Work out the finished part from the listing and answer in its coordinate system (mm). Round coordinates to 2 decimals unless told otherwise and drop trailing zeros. Write each loop counter-clockwise with the first axis right and the second up, starting at its lowest first coordinate (ties: lowest second). Pieces come first, ordered by that corner, then holes.
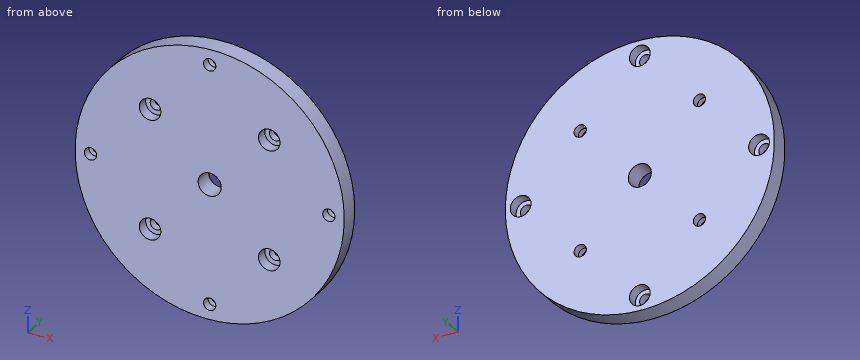
from build123d import *

# Parameters (mm, degrees)
SKETCH1_R           = 35
SKETCH1_R_2         = 3
BOSS_EXTRUDE1_DEPTH = 5
SKETCH2_R           = 1.6
CUT_EXTRUDE1_DEPTH  = 5
SKETCH4_R           = 2.8
SKETCH4_R_2         = 1.6
CUT_EXTRUDE2_DEPTH  = 3
SKETCH5_R           = 1.6
CUT_EXTRUDE3_DEPTH  = 10
SKETCH6_R           = 2.7
CUT_EXTRUDE4_DEPTH  = 2.8


with BuildPart() as part:
    # Sketch1 → Boss-Extrude1 (new body)
    with BuildSketch(Plane(origin=(0, 0, 0), x_dir=(1, 0, 0), z_dir=(0, 1, 0))):
        Circle(SKETCH1_R)
        Circle(SKETCH1_R_2, mode=Mode.SUBTRACT)
    extrude(amount=BOSS_EXTRUDE1_DEPTH)

    # Sketch2 → Cut-Extrude1 (cut)
    with BuildSketch(Plane.XZ):
        with Locations((15.5, 15.5)):
            Circle(SKETCH2_R)
        with Locations((15.5, -15.5)):
            Circle(SKETCH2_R)
        with Locations((-15.5, -15.5)):
            Circle(SKETCH2_R)
        with Locations((-15.5, 15.5)):
            Circle(SKETCH2_R)
    extrude(amount=-CUT_EXTRUDE1_DEPTH, mode=Mode.SUBTRACT)

    # Sketch4 → Cut-Extrude2 (cut)
    with BuildSketch(Plane.XZ):
        with Locations((-15.5, 15.5)):
            Circle(SKETCH4_R)
        with Locations((-15.5, 15.5)):
            Circle(SKETCH4_R_2, mode=Mode.SUBTRACT)
        with Locations((15.5, 15.5)):
            Circle(SKETCH4_R)
        with Locations((15.5, 15.5)):
            Circle(SKETCH4_R_2, mode=Mode.SUBTRACT)
        with Locations((15.5, -15.5)):
            Circle(SKETCH4_R)
        with Locations((15.5, -15.5)):
            Circle(SKETCH4_R_2, mode=Mode.SUBTRACT)
        with Locations((-15.5, -15.5)):
            Circle(SKETCH4_R)
        with Locations((-15.5, -15.5)):
            Circle(SKETCH4_R_2, mode=Mode.SUBTRACT)
    extrude(amount=-CUT_EXTRUDE2_DEPTH, mode=Mode.SUBTRACT)

    # Sketch5 → Cut-Extrude3 (cut)
    with BuildSketch(Plane(origin=(0, 5, 0), x_dir=(1, 0, 0), z_dir=(0, 1, 0))):
        with Locations((0, 31)):
            Circle(SKETCH5_R)
        with Locations((31, 0)):
            Circle(SKETCH5_R)
        with Locations((0, -31)):
            Circle(SKETCH5_R)
        with Locations((-31, 0)):
            Circle(SKETCH5_R)
    extrude(amount=-CUT_EXTRUDE3_DEPTH, mode=Mode.SUBTRACT)

    # Sketch6 → Cut-Extrude4 (cut)
    with BuildSketch(Plane(origin=(0, 5, 0), x_dir=(1, 0, 0), z_dir=(0, 1, 0))):
        with Locations((0, 31)):
            Circle(SKETCH6_R)
        with Locations((31, 0)):
            Circle(SKETCH6_R)
        with Locations((0, -31)):
            Circle(SKETCH6_R)
        with Locations((-31, 0)):
            Circle(SKETCH6_R)
    extrude(amount=-CUT_EXTRUDE4_DEPTH, mode=Mode.SUBTRACT)


solid = part.part
Q1. Find the intervals of material crossed by L1, parallel to Z at x = 0, y = 0.7; L2, parallel to Z at x = 0, y = 3.3; L3, parallel to Z at x = 16, y = 4.1, in increasing order.
Q2. Find section B-B (y = 3.8). Count the separate pieces of the cut face and the enclosed holes in it, plus the area to 3 significant figures.
Q3. Given pin 1 (1.5 mm diameter, centred on x = 8, y = 4, fed in from -Z); pin 2 (3 mm diameter, centred on y = 2.5, z = 11, fed in from -X); pin 3 (1.5 mm diameter, centred on y = 4, z = 11, fed in from -X), each flat-ended and moving along its own axis, determine where each tip first touches the part or whether it passes through.
Q4. Find section C-C (x = 15). Determine the outline of the cut face in (y, z) (3 decimals).
Q5. Find section A-A (z = 0). Determine the outline of the cut face in (x, y).
Q6. Find section D-D (x = -31). Determine the outline of the cut face in (y, z).
Report:
1. L1: z = -35 to -32.6, -29.4 to -3, 3 to 29.4, 32.6 to 35
1. L2: z = -35 to -33.7, -28.3 to -3, 3 to 28.3, 33.7 to 35
1. L3: z = -31.13 to -17.02, -13.98 to 13.98, 17.02 to 31.13
2. separate pieces: 1
2. enclosed holes: 9
2. area: 3,700 mm2
3. pin 1: stops at z = -34.24
3. pin 2: stops at x = -33.69
3. pin 3: stops at x = -33.47
4. outline: (0, -31.623) - (5, -31.623) - (5, -17.02) - (3, -17.02) - (3, -18.255) - (0, -18.255) - close; (0, -12.745) - (3, -12.745) - (3, -13.98) - (5, -13.98) - (5, 13.98) - (3, 13.98) - (3, 12.745) - (0, 12.745) - close; (0, 18.255) - (3, 18.255) - (3, 17.02) - (5, 17.02) - (5, 31.623) - (0, 31.623) - close
5. outline: (-35, 0) - (-32.6, 0) - (-32.6, 2.2) - (-33.7, 2.2) - (-33.7, 5) - (-35, 5) - close; (-29.4, 0) - (-3, 0) - (-3, 5) - (-28.3, 5) - (-28.3, 2.2) - (-29.4, 2.2) - close; (3, 0) - (29.4, 0) - (29.4, 2.2) - (28.3, 2.2) - (28.3, 5) - (3, 5) - close; (32.6, 0) - (35, 0) - (35, 5) - (33.7, 5) - (33.7, 2.2) - (32.6, 2.2) - close
6. outline: (0, -16.25) - (5, -16.25) - (5, -2.7) - (2.2, -2.7) - (2.2, -1.6) - (0, -1.6) - close; (0, 1.6) - (2.2, 1.6) - (2.2, 2.7) - (5, 2.7) - (5, 16.25) - (0, 16.25) - close
